from build123d import *

# Parameters (mm, degrees)
F2_R    = 1.27
F3_SIZE = 0.508
F4_R    = 1.27
F5_R    = 2.54
F6_R    = 2.54


with BuildPart() as f1:
    # F0 (on Front) → F1 (revolve)
    with BuildSketch(Plane.XZ):
        Polygon((6.35, 0), (6.35, 30.48), (11.43, 34.742626), (11.43, 48.26), (10.16, 48.26), (10.16, 35.334837), (5.08, 31.072211), (5.08, 1.27), (0, 1.27), (0, 0), align=None)
    revolve(axis=Axis((0, 0, 19.968925), (0, 0, -1)))

    # F2
    f2_edges = [f1.edges().sort_by_distance(p)[0] for p in [
        (-5.08, 0, 1.27),
    ]]
    fillet(f2_edges, radius=F2_R)

    # F3
    f3_edges = [f1.edges().sort_by_distance(p)[0] for p in [
        (-6.35, 0, 0),
    ]]
    chamfer(f3_edges, length=F3_SIZE)

    # F4
    f4_edges = [f1.edges().sort_by_distance(p)[0] for p in [
        (-6.35, 0, 30.48),
    ]]
    fillet(f4_edges, radius=F4_R)

    # F5
    f5_edges = [f1.edges().sort_by_distance(p)[0] for p in [
        (-11.43, 0, 34.742626),
    ]]
    fillet(f5_edges, radius=F5_R)

    # F6
    f6_edges = [f1.edges().sort_by_distance(p)[0] for p in [
        (-10.16, 0, 35.334837),
        (-5.08, 0, 31.072211),
    ]]
    fillet(f6_edges, radius=F6_R)


with BuildPart() as f7_1:
    # F7: copy of F1
    add(f1.part.moved(Location((69.85, 0, 0))))


solid = f1.part
Build history of the part. All positions in model axes, mm. A direction names the side the tool comes from. Round coordinates to 2 decimals unless told otherwise and drop trailing zeros. Order: outer loops, then holes, each group sorted by start corner. A loop starts at its lowest first (then second) coordinate and runs counter-clockwise, first axis right, second up. Notation, with made-up numbers: M 43.5,53.5 L 76.5,53.5 A14 cw 76.5,57.5 Z; hole C 66.25,-24.5 d4. An arc over 180 degrees is marked long. Use CSV: the item, a comma, the result in double quotes. Start each with the question number.
(1) Mould opens along X. For faces 3 (the face through (0, 0, 1.27)), 4 (the face through (0, 0, 0)), 5 (the face through (6.057, -1.907, 15.404)) say: +X half, -X half, draft (parallel to the pull), parting line (faces both ways), or undercut.
(2) Drill centre lines: probe 1 along Y at (x, z) = (0, 41.5); probe 2 along Y at (x, z) = (0, 21). Where is each one in solid material? Low to high.
(3) Tool access for faces 1 (the face through (9.69, -3.05, 42.31)), 2 (the face through (-8, 7, 48.26)): list every direction of +Z, -Z, +X, -X, +Y, -Y with a clear straight run to the whole face (end or side of a thin tool).
(4) Flat gauge pins, fed straight in: P1, Ø2, axis at x = -2, y = 8.5, coming from the -Z side; P2, Ø2.5, axis at x = 1.5, y = -1, coming from the +Z side; P3, Ø8, axis at y = -7.5, z = 18.5, coming from the -X side. Where does each tip first touch, or does it go through?
(5) Cut at B-B on z = 9.5. List the corners of the cut face in (x, y), then the cut area to 3 significant figures.
(6) Cut at A-A on z = 42.5. List the corners of the cut face in (x, y).
Findings:
1,face 3,"undercut"
1,face 4,"draft"
1,face 5,"parting line"
2,probe 1,"y = -11.43 to -10.16, 10.16 to 11.43"
2,probe 2,"y = -6.35 to -5.08, 5.08 to 6.35"
3,face 1,"+Z"
3,face 2,"+Z, +X, -X, +Y, -Y"
4,P1,"stops at z = 31.64"
4,P2,"stops at z = 1.27"
4,P3,"stops at x = -5.3"
5,outline,"C 0,0 d12.7; hole C 0,0 d10.16"
5,area,"45.6 mm^2"
6,outline,"C 0,0 d22.86; hole C 0,0 d20.32"
